For this review, use the dimensioned drawing (mm, ordinates from the lowest corner) and the shaded views. A direction names the side the tool comes from. Give positions to 0.01 mm unless a question says otherwise; leave off trailing zeros. Write each loop counter-clockwise with the first axis right and the second up, starting at its lowest first coordinate (ties: lowest second). Pieces come first, ordered by that corner, then holes.
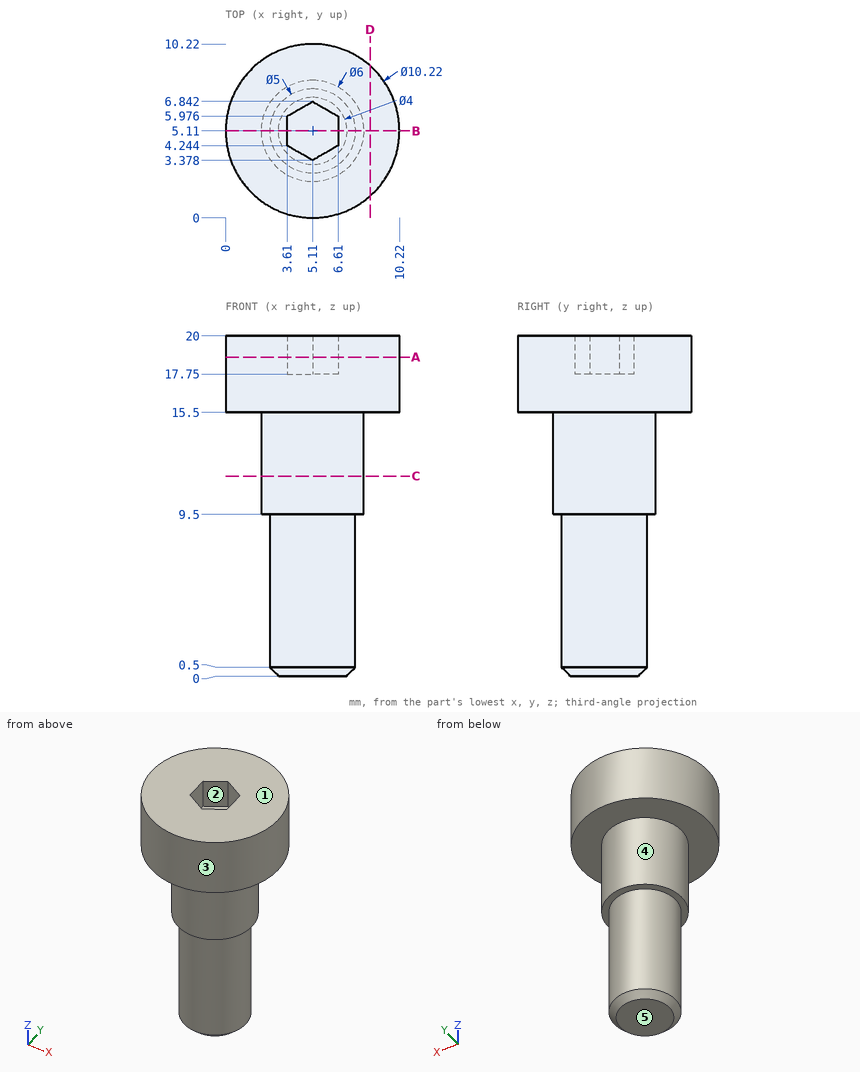
(1) We need section B-B (y = 5.11). Write out the cut boundary in (x, z).
(2) Tool access review of the marked faces 4 and 5: name each direction out of +Z, -Z, +X, -X, +Y, -Y from which nothing blocks a thin tool from reaching the whole face with its end or side.
(3) We need section A-A (z = 18.75). Write out the cut boundary in (x, y), and give its area (3 significant figures).
(4) For L1, parallel to X at y = 5, z = 16; L2, parallel to Z at x = 2, y = 1.75; L3, parallel to Z at x = 5.25, y = 6.5, list the stretches that pass through material, from the lowest coordinate up.
(5) We need section C-C (z = 11.75). Write out the cut boundary in (x, y), and give its area (3 significant figures).
(6) The part is to be moulded in two halves that separate along X. For the marked faces 1, 2 and 3, say which applies: +X half, -X half, draft (parallel to the pull), parting line (faces both ways), or undercut.
(7) Clearance check with flat-ended pins moving along their axes: pin 1 Ø6 at (x, z) = (3, 13) entering from -Y; pin 2 Ø4 at (x, z) = (5.5, 8.5) entering from -Y; pin 3 Ø4 at (y, z) = (7.5, 12) entering from +X. State where each tip first meets the part, or that it passes through.
(8) We need section D-D (x = 8.5). Write out the cut boundary in (y, z), and give its area (3 significant figures).
The answers:
1. outline: (0, 15.5) - (2.11, 15.5) - (2.11, 9.5) - (2.61, 9.5) - (2.61, 0.5) - (3.11, 0) - (7.11, 0) - (7.61, 0.5) - (7.61, 9.5) - (8.11, 9.5) - (8.11, 15.5) - (10.22, 15.5) - (10.22, 20) - (6.61, 20) - (6.61, 17.75) - (3.61, 17.75) - (3.61, 20) - (0, 20) - close
2. face 4: -Z
2. face 5: -Z, +X, -X, +Y, -Y
3. outline: circle Ø10.22 at (5.11, 5.11); hole (3.61, 4.24) - (5.11, 3.38) - (6.61, 4.24) - (6.61, 5.98) - (5.11, 6.84) - (3.61, 5.98) - close
3. area: 74.2 mm2
4. L1: x = 0 to 10.22
4. L2: z = 15.5 to 20
4. L3: z = 0 to 17.75
5. outline: circle Ø6 at (5.11, 5.11)
5. area: 28.3 mm2
6. face 1: draft
6. face 2: undercut
6. face 3: parting line
7. pin 1: stops at y = 0.02
7. pin 2: stops at y = 2.11
7. pin 3: stops at x = 8.08
8. outline: (1.29, 15.5) - (8.93, 15.5) - (8.93, 20) - (1.29, 20) - close
8. area: 34.4 mm2
